Could you check a few things on this drawing? It's one solid part, dimensions in mm from its lowest x, y, z. A direction names the side the tool comes from. Give positions to 0.01 mm unless a question says otherwise; leave off trailing zeros. Order: outer loops, then holes, each group sorted by start corner. A loop starts at its lowest first (then second) coordinate and runs counter-clockwise, first axis right, second up.
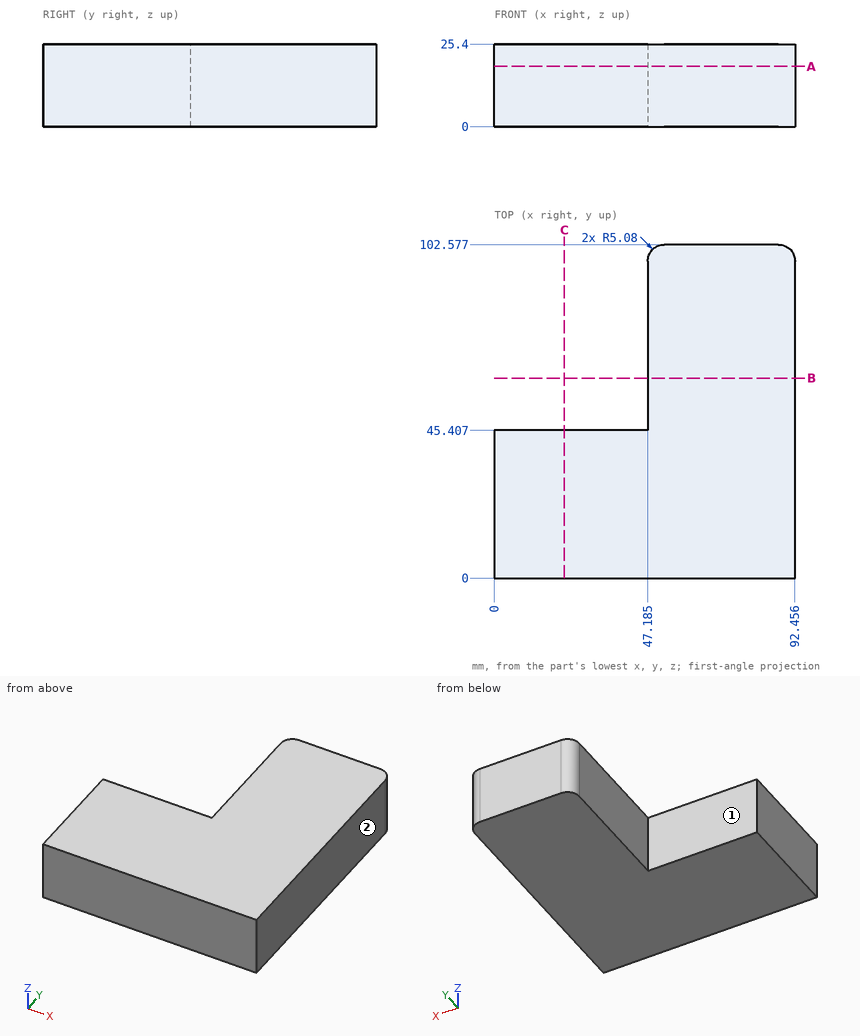
Item 1: For the marked faces 1 and 2, which set-ups out of +Z, -Z, +X, -X, +Y, -Y let a thin tool reach every point of the face, with its end or its side?
Findings:
face 1: +Z, -Z, -X, +Y
face 2: +Z, -Z, +X, +Y, -Y
Item 2: Please list where these lines run through material, in increasing order: line 1 along Y through (x, z) = (14.5, 19.25); line 2 along X through (y, z) = (60, 24.25) (1 decimal); line 3 along Y through (x, z) = (52, 9).
Findings:
line 1: y = 0 to 45.41
line 2: x = 47.2 to 92.5
line 3: y = 0 to 102.57
Item 3: For pin 1 (12.5 mm diameter, centred on y = 81, z = 7.5, fed in from -X) (1 decimal); pin 2 (3 mm diameter, centred on x = 14, z = 11, fed in from +Y), each with a flat end and sliding along its axis, tell me the tip position at first contact or that it passes through.
Findings:
pin 1: stops at x = 47.2
pin 2: stops at y = 45.41
Item 4: Imagine slicing it at A-A on z = 18.5. List the corners of the cut face in (x, y) for me (1 decimal).
Findings:
outline: (0, 0) - (92.5, 0) - (92.5, 97.5) arc R5.1 ccw to (87.4, 102.6) - (52.3, 102.6) arc R5.1 ccw to (47.2, 97.5) - (47.2, 45.4) - (0, 45.4) - close
Item 5: Imagine slicing it at B-B on y = 61.5. List the corners of the cut face in (x, z) for me (1 decimal), then the cut area to 3 significant figures.
Findings:
outline: (47.2, 0) - (92.5, 0) - (92.5, 25.4) - (47.2, 25.4) - close
area: 1,150 mm2
Item 6: Imagine slicing it at C-C on x = 21.5. List the corners of the cut face in (y, z) for me.
Findings:
outline: (0, 0) - (45.41, 0) - (45.41, 25.4) - (0, 25.4) - close
